```python
from build123d import *

# Parameters (mm, degrees)
EXTRUDE_1_DEPTH = 0.6


with BuildPart() as part:
    # 스케치1 → 보스-돌출1 (new body)
    with BuildSketch(Plane.XY):
        with BuildLine():
            ThreePointArc((4.243865228, 6.118140931), (3.92164821, 5.921191263), (3.601804057, 5.720411047))
            ThreePointArc((3.601804057, 5.720411047), (3.493384012, 5.24542324), (3.316336948, 4.791526049))
            ThreePointArc((3.316336948, 4.791526049), (2.452686661, 4.097818684), (1.509336268, 3.517119312))
            ThreePointArc((1.509336268, 3.517119312), (2.704109532, 3.767922564), (3.790546418, 4.324735205))
            ThreePointArc((3.790546418, 4.324735205), (4.007319334, 4.893950514), (4.243865228, 5.455237077))
            ThreePointArc((4.243865228, 5.455237077), (4.639299082, 5.669042259), (5.043553271, 5.865661533))
            ThreePointArc((5.043553271, 5.865661533), (5.086534646, 4.510854203), (5.043553271, 3.156046874))
            ThreePointArc((5.043553271, 3.156046874), (6.065944614, -0.097812915), (5.291753627, -3.419486575))
            ThreePointArc((5.291753627, -3.419486575), (3.490836657, -9.120276828), (-0.418085028, -13.643842092))
            ThreePointArc((-0.418085028, -13.643842092), (-2.087490816, -14.704669315), (-3.875685356, -15.550027444))
            ThreePointArc((-3.875685356, -15.550027444), (-4.814989199, -15.5684183), (-5.740747963, -15.728420312))
            ThreePointArc((-5.740747963, -15.728420312), (-6.513490531, -15.594064313), (-7.296832392, -15.633537604))
            ThreePointArc((-7.296832392, -15.633537604), (-7.368791385, -14.902567754), (-7.494700457, -14.178936686))
            ThreePointArc((-7.494700457, -14.178936686), (-8.304954519, -13.843397992), (-9.155598119, -14.056713079))
            ThreePointArc((-9.155598119, -14.056713079), (-8.9873833, -14.884534295), (-8.949428325, -15.728420312))
            ThreePointArc((-8.949428325, -15.728420312), (-12.316982906, -16.443277918), (-15.620992713, -17.410213517))
            ThreePointArc((-15.620992713, -17.410213517), (-18.192390504, -20.114679115), (-21.053078027, -22.511069665))
            ThreePointArc((-21.053078027, -22.511069665), (-22.181356159, -23.04421905), (-23.359176817, -23.456527561))
            ThreePointArc((-23.359176817, -23.456527561), (-21.55820937, -20.881039072), (-19.369361534, -18.625918265))
            ThreePointArc((-19.369361534, -18.625918265), (-13.849484699, -12.644014904), (-8.593743971, -6.428759681))
            ThreePointArc((-8.593743971, -6.428759681), (-6.650317937, -5.116178912), (-5.664079914, -2.988478841))
            ThreePointArc((-5.664079914, -2.988478841), (-6.968956966, -4.648017071), (-8.787254134, -5.720661777))
            ThreePointArc((-8.787254134, -5.720661777), (-14.217270083, -11.359132573), (-19.298032623, -17.314237787))
            ThreePointArc((-19.298032623, -17.314237787), (-20.952003277, -18.09423566), (-22.701668736, -18.625918265))
            ThreePointArc((-22.701668736, -18.625918265), (-20.032240522, -15.856920342), (-16.99977962, -13.491042629))
            ThreePointArc((-16.99977962, -13.491042629), (-16.716409139, -12.979319841), (-16.386941379, -12.49598762))
            ThreePointArc((-16.386941379, -12.49598762), (-15.418772116, -10.250862917), (-14.374813618, -8.039960994))
            ThreePointArc((-14.374813618, -8.039960994), (-11.420678404, -2.410213973), (-7.380723905, 2.498934021))
            ThreePointArc((-7.380723905, 2.498934021), (-6.377004033, 4.393223264), (-5.210202068, 6.191655495))
            ThreePointArc((-5.210202068, 6.191655495), (-1.978219396, 9.037163181), (2.318833307, 9.316383632))
            ThreePointArc((2.318833307, 9.316383632), (3.338100738, 8.829609856), (4.243865228, 8.154742835))
            ThreePointArc((4.243865228, 8.154742835), (3.456899221, 7.145606029), (2.786183745, 6.055737532))
            ThreePointArc((2.786183745, 6.055737532), (3.51538621, 6.078489728), (4.243865228, 6.118140931))
        make_face()
        with BuildLine():
            ThreePointArc((-2.808227805, 1.460594831), (-5.951081989, -1.825237175), (-8.949428325, -5.243444841))
            ThreePointArc((-8.949428325, -5.243444841), (-8.831818054, -5.27564433), (-8.711437416, -5.295073305))
            ThreePointArc((-8.711437416, -5.295073305), (-5.278864783, -2.182820323), (-1.91601492, 1.004641725))
            ThreePointArc((-1.91601492, 1.004641725), (-2.267690382, 1.417401617), (-2.808227805, 1.460594831))
        make_face(mode=Mode.SUBTRACT)
        with BuildLine():
            ThreePointArc((-0.993904208, 6.118140931), (-0.547936142, 6.833647448), (0.215079605, 7.192317298))
            ThreePointArc((0.215079605, 7.192317298), (0.841318807, 7.133240086), (1.361301437, 6.779285683))
            ThreePointArc((1.361301437, 6.779285683), (1.548522148, 6.776978051), (1.702780334, 6.670858627))
            ThreePointArc((1.702780334, 6.670858627), (0.955764837, 5.731971759), (-0.237955168, 5.611252025))
            ThreePointArc((-0.237955168, 5.611252025), (-0.653261747, 5.809021292), (-0.993904208, 6.118140931))
        make_face(mode=Mode.SUBTRACT)
    extrude(amount=EXTRUDE_1_DEPTH)


solid = part.part
```
Geometry: final body of the model. Coordinates: model frame, mm. A direction names the side the tool comes from. Round coordinates to 2 decimals unless told otherwise and drop trailing zeros. Write each loop counter-clockwise with the first axis right and the second up, starting at its lowest first coordinate (ties: lowest second). Pieces come first, ordered by that corner, then holes.
Item 1: Section query D-D (z = 0.25). Give the number of separate pieces and of enclosed holes in the cut face, plus the area to 3 significant figures.
Item 2: Section query B-B (y = -4.5). Return loops of the section in (x, z), plus the area to 3 significant figures.
Item 3: Section query A-A (y = -9). Return loops of the section in (x, z), plus the area to 3 significant figures.
Item 4: Pin query (flat end, axial travel): P1, Ø1, axis at x = -6.5, y = 6, coming from the -Z side. Return the tip coordinate at first contact, or that it passes through.
Item 5: Mould query, pull axis X, two halves, no side actions, for faces 1 (the face through (-5.91, -1.78, 0.3)), 2 (the face through (3.53, -9.05, 0.3)), 3 (the face through (-5, -7, 0.6)), 4 (the face through (-11.47, -2.485, 0.296)). Classes: +X half, -X half, draft (parallel to the pull), parting line (faces both ways), or undercut.
Item 6: Section query C-C (x = 1). Return loops of the section in (y, z).
Item 7: Set-up query: faces 5 (the face through (-20.928, -18.085, 0.296)), 6 (the face through (-18.154, -20.079, 0.296)). Return all of +Z, -Z, +X, -X, +Y, -Y with unobstructed straight access to the full face (end or side cutting, diameter ignored); none if empty.
Item 8: Material intervals for L1, parallel to Y at x = 3.75, z = 0.1; L2, parallel to X at y = -15, z = 0.4; L3, parallel to X at y = 6, z = 0.45, sorted ascending.
Completed:
1. separate pieces: 1
1. enclosed holes: 2
1. area: 373 mm2
2. outline: (-12.69, 0) - (-8.32, 0) - (-8.32, 0.6) - (-12.69, 0.6) - close; (-7.82, 0) - (-6.81, 0) - (-6.81, 0.6) - (-7.82, 0.6) - close; (-6.21, 0) - (5.14, 0) - (5.14, 0.6) - (-6.21, 0.6) - close
2. area: 10.0 mm2
3. outline: (-14.84, 0) - (-12.02, 0) - (-12.02, 0.6) - (-14.84, 0.6) - close; (-10.71, 0) - (3.56, 0) - (3.56, 0.6) - (-10.71, 0.6) - close
3. area: 10.3 mm2
4. P1: passes through
5. face 1: undercut
5. face 2: +X half
5. face 3: draft
5. face 4: -X half
6. outline: (-12.4, 0) - (5.76, 0) - (5.76, 0.6) - (-12.4, 0.6) - close; (7.06, 0) - (9.53, 0) - (9.53, 0.6) - (7.06, 0.6) - close
7. face 5: +Z, -Z
7. face 6: +Z, -Z, +X, -Y
8. L1: y = -8.64 to 4.3, 5.81 to 6.09, 7.55 to 8.56
8. L2: x = -19.03 to -17.4, -15.97 to -8.97, -7.36 to -2.65
8. L3: x = -5.35 to -0.89, 1.31 to 4.05
